For this review, take the finished solid that the model builds, in its own axes (mm). Face numbers are marked on the shaded views. A direction names the side the tool comes from. Coordinates: 2 decimals unless noted, no trailing zeros. Write each loop counter-clockwise with the first axis right and the second up, starting at its lowest first coordinate (ties: lowest second). Pieces come first, ordered by that corner, then holes.
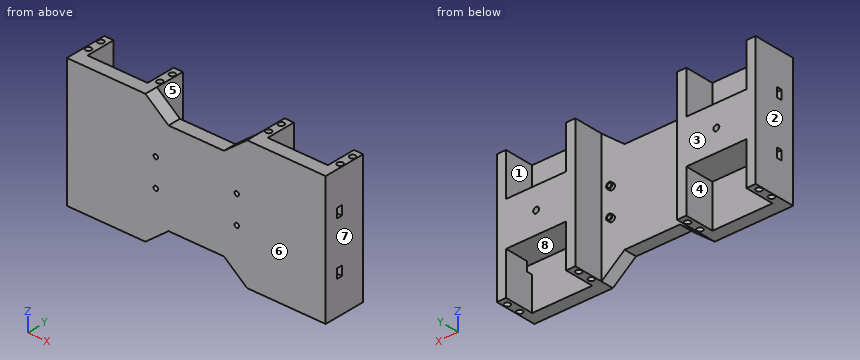
```python
from build123d import *

# Parameters (mm, degrees)
SKETCH2_W           = 41.275
SKETCH2_H           = 29.464
BOSS_EXTRUDE1_DEPTH = 8.89
BOSS_EXTRUDE2_DEPTH = 29.14396
SKETCH6_R           = 2
CUT_EXTRUDE1_DEPTH  = 6.5
SKETCH7_R           = 2
CUT_EXTRUDE2_DEPTH  = 6
SKETCH8_R           = 2.135
SKETCH8_R_2         = 1.5
EXTRUDE_THIN1_DEPTH = 2
CUT_EXTRUDE3_START  = -21.78
SKETCH8_3_R         = 1.5
CUT_EXTRUDE3_DEPTH  = 21.78
CUT_EXTRUDE4_START  = -82.9
SKETCH7_2_R         = 2
CUT_EXTRUDE4_DEPTH  = 6
SKETCH9_W           = 6.35
SKETCH9_H           = 3.81
CUT_EXTRUDE5_DEPTH  = 6.35
CUT_EXTRUDE6_START  = -177.8
SKETCH9_2_W         = 6.35
SKETCH9_2_H         = 3.81
CUT_EXTRUDE6_DEPTH  = 6.35


with BuildPart() as part:
    # Sketch2 → Boss-Extrude1 (new body)
    with BuildSketch(Plane(origin=(0, 0, 0), x_dir=(1, 0, 0), z_dir=(0, 1, 0))):
        with Locations((26.9875, 74.168)):
            Rectangle(SKETCH2_W, SKETCH2_H)
        with Locations((26.9875, 14.732)):
            Rectangle(SKETCH2_W, SKETCH2_H)
        Polygon((0, 88.9), (0, 0), (6.35, 0), (6.35, 29.464), (47.625, 29.464), (47.625, 0), (53.975, 0), (53.975, 12.7), (53.975, 76.2), (53.975, 88.9), (47.625, 88.9), (47.625, 59.436), (6.35, 59.436), (6.35, 88.9), align=None)
        Polygon((53.975, 12.7), (69.85, 12.7), (107.95, 12.7), (123.825, 12.7), (123.825, 76.2), (107.95, 76.2), (69.85, 76.2), (53.975, 76.2), align=None)
        Polygon((53.975, 12.7), (53.975, 0), (69.85, 12.7), align=None)
        Polygon((107.95, 12.7), (123.825, 0), (123.825, 12.7), align=None)
        Polygon((123.825, 12.7), (123.825, 0), (130.175, 0), (130.175, 29.464), (171.45, 29.464), (171.45, 0), (177.8, 0), (177.8, 88.9), (171.45, 88.9), (171.45, 59.436), (130.175, 59.436), (130.175, 88.9), (123.825, 88.9), (123.825, 76.2), align=None)
        with Locations((150.8125, 14.732)):
            Rectangle(SKETCH2_W, SKETCH2_H)
        with Locations((150.8125, 74.168)):
            Rectangle(SKETCH2_W, SKETCH2_H)
        Polygon((123.825, 76.2), (123.825, 88.9), (107.95, 76.2), align=None)
        Polygon((69.85, 76.2), (53.975, 88.9), (53.975, 76.2), align=None)
    extrude(amount=BOSS_EXTRUDE1_DEPTH)

    # Sketch2<3> → Boss-Extrude2 (add)
    with BuildSketch(Plane(origin=(0, 0, 0), x_dir=(1, 0, 0), z_dir=(0, 1, 0))):
        Polygon((0, 88.9), (0, 0), (6.35, 0), (6.35, 29.464), (47.625, 29.464), (47.625, 0), (53.975, 0), (53.975, 12.7), (53.975, 76.2), (53.975, 88.9), (47.625, 88.9), (47.625, 59.436), (6.35, 59.436), (6.35, 88.9), align=None)
        Polygon((123.825, 12.7), (123.825, 0), (130.175, 0), (130.175, 29.464), (171.45, 29.464), (171.45, 0), (177.8, 0), (177.8, 88.9), (171.45, 88.9), (171.45, 59.436), (130.175, 59.436), (130.175, 88.9), (123.825, 88.9), (123.825, 76.2), align=None)
    extrude(amount=BOSS_EXTRUDE2_DEPTH)

    # Sketch6 → Cut-Extrude1 (cut)
    with BuildSketch(Plane(origin=(0, 29.14396, 0), x_dir=(1, 0, 0), z_dir=(0, 1, 0))):
        with Locations(Location((26.9875, 44.45, 0), (0, 0, 270))):
            Circle(SKETCH6_R)
        with Locations(Location((150.8125, 44.45, 0), (0, 0, 270))):
            Circle(SKETCH6_R)
    extrude(amount=-CUT_EXTRUDE1_DEPTH, mode=Mode.SUBTRACT)

    # Sketch7 → Cut-Extrude2 (cut)
    with BuildSketch(Plane.XY):
        with Locations((2.4375, 14.04)):
            Circle(SKETCH7_R)
        with Locations((51.5375, 14.04)):
            Circle(SKETCH7_R)
        with Locations((2.4375, 23.740006)):
            Circle(SKETCH7_R)
        with Locations((51.5375, 23.740006)):
            Circle(SKETCH7_R)
        with Locations(Location((126.2625, 23.740006, 0), (0, 0, 180))):
            Circle(SKETCH7_R)
        with Locations(Location((175.3625, 23.740006, 0), (0, 0, 180))):
            Circle(SKETCH7_R)
        with Locations(Location((126.2625, 14.04, 0), (0, 0, 180))):
            Circle(SKETCH7_R)
        with Locations(Location((175.3625, 14.04, 0), (0, 0, 180))):
            Circle(SKETCH7_R)
    extrude(amount=-CUT_EXTRUDE2_DEPTH, mode=Mode.SUBTRACT)

    # Sketch8 → Extrude-Thin1 (add)
    # profile 1 of 4: a face of its own
    with BuildSketch(Plane(origin=(0, 8.89, 0), x_dir=(1, 0, 0), z_dir=(0, 1, 0))):
        with Locations((61.087, 53.975)):
            Circle(SKETCH8_R)
        with Locations((61.087, 53.975)):
            Circle(SKETCH8_R_2, mode=Mode.SUBTRACT)
    # profile 2 of 4: a face of its own
    with BuildSketch(Plane(origin=(0, 8.89, 0), x_dir=(1, 0, 0), z_dir=(0, 1, 0))):
        with Locations((61.087, 34.925)):
            Circle(SKETCH8_R)
        with Locations((61.087, 34.925)):
            Circle(SKETCH8_R_2, mode=Mode.SUBTRACT)
    # profile 3 of 4: a face of its own
    with BuildSketch(Plane(origin=(0, 8.89, 0), x_dir=(1, 0, 0), z_dir=(0, 1, 0))):
        with Locations((116.713, 34.925)):
            Circle(SKETCH8_R)
        with Locations((116.713, 34.925)):
            Circle(SKETCH8_R_2, mode=Mode.SUBTRACT)
    # profile 4 of 4: a face of its own
    with BuildSketch(Plane(origin=(0, 8.89, 0), x_dir=(1, 0, 0), z_dir=(0, 1, 0))):
        with Locations((116.713, 53.975)):
            Circle(SKETCH8_R)
        with Locations((116.713, 53.975)):
            Circle(SKETCH8_R_2, mode=Mode.SUBTRACT)
    extrude(amount=EXTRUDE_THIN1_DEPTH)

    # Sketch8<3> → Cut-Extrude3 (cut)
    with BuildSketch(Plane(origin=(0, 8.89, 0), x_dir=(1, 0, 0), z_dir=(0, 1, 0)).offset(CUT_EXTRUDE3_START)):
        with Locations(Location((61.087, 53.975, 0), (0, 0, 270))):
            Circle(SKETCH8_3_R)
        with Locations(Location((61.087, 34.925, 0), (0, 0, 270))):
            Circle(SKETCH8_3_R)
        with Locations(Location((116.713, 34.925, 0), (0, 0, 270))):
            Circle(SKETCH8_3_R)
        with Locations(Location((116.713, 53.975, 0), (0, 0, 270))):
            Circle(SKETCH8_3_R)
    extrude(amount=CUT_EXTRUDE3_DEPTH, mode=Mode.SUBTRACT)

    # Sketch7<2> → Cut-Extrude4 (cut)
    with BuildSketch(Plane.XY.offset(CUT_EXTRUDE4_START)):
        with Locations((2.4375, 14.04)):
            Circle(SKETCH7_2_R)
        with Locations((51.5375, 14.04)):
            Circle(SKETCH7_2_R)
        with Locations((2.4375, 23.740006)):
            Circle(SKETCH7_2_R)
        with Locations((51.5375, 23.740006)):
            Circle(SKETCH7_2_R)
        with Locations(Location((126.2625, 23.740006, 0), (0, 0, 180))):
            Circle(SKETCH7_2_R)
        with Locations(Location((175.3625, 23.740006, 0), (0, 0, 180))):
            Circle(SKETCH7_2_R)
        with Locations(Location((126.2625, 14.04, 0), (0, 0, 180))):
            Circle(SKETCH7_2_R)
        with Locations(Location((175.3625, 14.04, 0), (0, 0, 180))):
            Circle(SKETCH7_2_R)
    extrude(amount=-CUT_EXTRUDE4_DEPTH, mode=Mode.SUBTRACT)

    # Sketch9 → Cut-Extrude5 (cut)
    with BuildSketch(Plane.ZY):
        with Locations((-26.289, 10.795)):
            Rectangle(SKETCH9_W, SKETCH9_H)
        with Locations((-62.611, 10.795)):
            Rectangle(SKETCH9_W, SKETCH9_H)
    extrude(amount=-CUT_EXTRUDE5_DEPTH, mode=Mode.SUBTRACT)

    # Sketch9<2> → Cut-Extrude6 (cut)
    with BuildSketch(Plane.ZY.offset(CUT_EXTRUDE6_START)):
        with Locations((-26.289, 10.795)):
            Rectangle(SKETCH9_2_W, SKETCH9_2_H)
        with Locations((-62.611, 10.795)):
            Rectangle(SKETCH9_2_W, SKETCH9_2_H)
    extrude(amount=CUT_EXTRUDE6_DEPTH, mode=Mode.SUBTRACT)


solid = part.part
```
Q1. Add section B-B (z = -44.45). State the section outline as (x, y) points (1 decimal).
Ans:
outline: (0, 0) - (177.8, 0) - (177.8, 29.1) - (152.8, 29.1) - (152.8, 22.6) - (148.8, 22.6) - (148.8, 29.1) - (123.8, 29.1) - (123.8, 8.9) - (54, 8.9) - (54, 29.1) - (29, 29.1) - (29, 22.6) - (25, 22.6) - (25, 29.1) - (0, 29.1) - close
Q2. Draft analysis for pull direction X (two halves, no side actions). For the marked faces 6, 7 and 8, state which applies: +X half, -X half, draft (parallel to the pull), parting line (faces both ways), or undercut.
Ans:
face 6: draft
face 7: +X half
face 8: undercut
Q3. Add section C-C (y = 6). State the section outline as (x, z) points (3 decimals).
Ans:
outline: (0, -88.9) - (53.975, -88.9) - (69.85, -76.2) - (107.95, -76.2) - (123.825, -88.9) - (177.8, -88.9) - (177.8, 0) - (123.825, 0) - (107.95, -12.7) - (69.85, -12.7) - (53.975, 0) - (0, 0) - close; hole circle Ø3 at (61.087, -53.975); hole circle Ø3 at (61.087, -34.925); hole circle Ø3 at (116.713, -53.975); hole circle Ø3 at (116.713, -34.925)
Q4. Add section D-D (z = -74). State the section outline as (x, y) points (3 decimals), then the cut area to 3 significant figures.
Ans:
outline: (0, 0) - (177.8, 0) - (177.8, 29.144) - (171.45, 29.144) - (171.45, 8.89) - (130.175, 8.89) - (130.175, 29.144) - (123.825, 29.144) - (123.825, 8.89) - (53.975, 8.89) - (53.975, 29.144) - (47.625, 29.144) - (47.625, 8.89) - (6.35, 8.89) - (6.35, 29.144) - (0, 29.144) - close
area: 2,100 mm2
Q5. For probe 1 along X at (y, z) = (23.75, -16) (3 decimals); probe 2 along X at (y, z) = (23, -51.5) (3 decimals), list the stretches that pass through material, from the lowest coordinate up.
Ans:
probe 1: x = 0 to 6.35, 47.625 to 53.975, 123.825 to 130.175, 171.45 to 177.8
probe 2: x = 0 to 53.975, 123.825 to 177.8
Q6. Clearance check with flat-ended pins moving along their axes: pin 1 Ø4.5 at (x, y) = (50.5, 14.5) entering from -Z; pin 2 Ø6 at (x, y) = (163, 23.5) entering from -Z; pin 3 Ø21 at (x, z) = (94.5, -62) entering from +Y; pin 4 Ø8 at (x, y) = (89.5, 3.5) entering from -Z. State where each tip first meets the part, or that it passes through.
Ans:
pin 1: stops at z = -88.9
pin 2: stops at z = -59.44
pin 3: stops at y = 8.89
pin 4: stops at z = -76.2
Q7. Add section A-A (x = 17.5). State the section outline as (y, z) points.
Ans:
outline: (0, -88.9) - (8.89, -88.9) - (8.89, -59.44) - (29.14, -59.44) - (29.14, -29.46) - (8.89, -29.46) - (8.89, 0) - (0, 0) - close
Q8. Tool access review of the marked faces 1, 2, 3, 4 and 5: name each direction out of +Z, -Z, +X, -X, +Y, -Y from which nothing blocks a thin tool from reaching the whole face with its end or side.
Ans:
face 1: +Z, +Y
face 2: +Z, -Z, -X, +Y, -Y
face 3: +Z, -Z, +X, -X, +Y
face 4: -Z, +Y
face 5: +Z, -Z, +Y
